from build123d import *

# Parameters (mm, degrees)
SKETCH1_R           = 2
SKETCH1_W           = 5
SKETCH1_H           = 5
BOSS_EXTRUDE7_DEPTH = 5
FILLET2_R           = 3


with BuildPart() as part:
    # Sketch1 → Boss-Extrude7 (new body)
    with BuildSketch(Plane(origin=(0, 0, 0), x_dir=(1, 0, 0), z_dir=(0, 1, 0))):
        Polygon((-29.056186132, 30.501621615), (-21.556186132, 30.501621615), (-21.556186132, 35.501621615), (-16.556186132, 35.501621615), (-16.556186132, 30.501621615), (-13.556186132, 30.501621615), (-13.556186132, 27.501621615), (-15.056186132, 27.501621615), (-15.056186132, 25.001621615), (-13.556186132, 25.001621615), (-13.556186132, 20.501621615), (-9.556186132, 20.501621615), (-9.556186132, 25.001621615), (-8.056186132, 25.001621615), (-8.056186132, 27.501621615), (-9.556186132, 27.501621615), (-9.556186132, 30.501621615), (-6.556186132, 30.501621615), (-6.556186132, 35.501621615), (-1.556186132, 35.501621615), (-1.556186132, 30.501621615), (5.943813868, 30.501621615), (5.943813868, -74.498378385), (-29.056186132, -74.498378385), align=None)
        with Locations(Location((0.443813868, 10.501621615, 0), (0, 0, 270))):
            Circle(SKETCH1_R, mode=Mode.SUBTRACT)
        with Locations(Location((-23.556186132, 10.501621615, 0), (0, 0, 90))):
            Circle(SKETCH1_R, mode=Mode.SUBTRACT)
        with Locations(Location((0.443813868, -46.498378385, 0), (0, 0, 90))):
            Circle(SKETCH1_R, mode=Mode.SUBTRACT)
        with Locations(Location((-23.556186132, -46.498378385, 0), (0, 0, 270))):
            Circle(SKETCH1_R, mode=Mode.SUBTRACT)
        with Locations(Location((-11.556186132, -68.998378385, 0), (0, 0, 270))):
            Circle(SKETCH1_R, mode=Mode.SUBTRACT)
        with Locations((-23.556186132, 3.001621615)):
            Rectangle(SKETCH1_W, SKETCH1_H, mode=Mode.SUBTRACT)
        with Locations((-23.556186132, 18.001621615)):
            Rectangle(SKETCH1_W, SKETCH1_H, mode=Mode.SUBTRACT)
        with Locations((0.443813868, 3.001621615)):
            Rectangle(SKETCH1_W, SKETCH1_H, mode=Mode.SUBTRACT)
        with Locations((0.443813868, 18.001621615)):
            Rectangle(SKETCH1_W, SKETCH1_H, mode=Mode.SUBTRACT)
        with Locations((0.443813868, -38.998378385)):
            Rectangle(SKETCH1_W, SKETCH1_H, mode=Mode.SUBTRACT)
        with Locations((0.443813868, -53.998378385)):
            Rectangle(SKETCH1_W, SKETCH1_H, mode=Mode.SUBTRACT)
        with Locations((-23.556186132, -53.998378385)):
            Rectangle(SKETCH1_W, SKETCH1_H, mode=Mode.SUBTRACT)
        with Locations((-23.556186132, -38.998378385)):
            Rectangle(SKETCH1_W, SKETCH1_H, mode=Mode.SUBTRACT)
        with Locations((-19.056186132, -68.998378385)):
            Rectangle(SKETCH1_W, SKETCH1_H, mode=Mode.SUBTRACT)
        with Locations((-4.056186132, -68.998378385)):
            Rectangle(SKETCH1_W, SKETCH1_H, mode=Mode.SUBTRACT)
    extrude(amount=BOSS_EXTRUDE7_DEPTH)

    # Fillet2
    fillet2_edges = [part.edges().sort_by_distance(p)[0] for p in [
        (5.943813868, 2.5, 74.498378385),
        (-29.056186132, 2.5, 74.498378385),
    ]]
    fillet(fillet2_edges, radius=FILLET2_R)


solid = part.part
Verification items for the finished model (mm, model axes). A direction names the side the tool comes from. Give positions to 0.01 mm unless a question says otherwise; leave off trailing zeros. Write each loop counter-clockwise with the first axis right and the second up, starting at its lowest first coordinate (ties: lowest second). Pieces come first, ordered by that corner, then holes. Notation, with made-up numbers: M 37,-19 L 61,-19 A22 ccw 61,20 Z; hole C -22.5,72.5 d2. An arc over 180 degrees is marked long. Put each result on its own line as item: value. Start each with the question number.
1. Scan lines: line 1 along Z through (x, y) = (-26, 1.7); line 2 along X through (y, z) = (1.85, -5); line 3 along Z through (x, y) = (-6.5, 0.75). Record each from-to range of solid material in increasing order. Write a range as [from, to].
2. Draft check along X on faces 4 (the face through (-25, 2, -30.502)), 5 (the face through (-21.556, 2, -33)), 6 (the face through (-26.056, 2, -3)). Enter one of: +X half, -X half, draft (parallel to the pull), parting line (faces both ways), or undercut.
3. Set-up check for faces 1 (the face through (-4, 2, -35.502)), 2 (the face through (-12, 2, -20.502)), 3 (the face through (-24, 2, -20.502)): record each of +Z, -Z, +X, -X, +Y, -Y from which the full face is reachable in a straight line by a thin tool's end or side.
4. Go/stop test with flat-tipped pins: pin 1 Ø2.5 at (x, y) = (-8.5, 2.5) entering from -Z; pin 2 Ø1.2 at (x, y) = (-11, 3.5) entering from -Z. Record where each tip stops, or that it passes through.
5. Section check A-A (z = 38.5). Record the cut outline in (x, y).
6. Section check B-B (y = 3.95). Give the number of separate pieces and of enclosed holes in the cut face, and give its area (3 significant figures).
Answer list:
1. line 1: [-30.5, -20.5], [-15.5, -5.5], [-0.5, 36.5], [41.5, 51.5], [56.5, 74.5]
1. line 2: [-29.06, -26.06], [-21.06, -2.06], [2.94, 5.94]
1. line 3: [-35.5, 66.5], [71.5, 74.5]
2. face 4: draft
2. face 5: -X half
2. face 6: undercut
3. face 1: -Z, +X, -X, +Y, -Y
3. face 2: -Z, +Y, -Y
3. face 3: +Y, -Y
4. pin 1: z = -30.5
4. pin 2: z = -20.5
5. outline: M -29.06,0 L -26.06,0 L -26.06,5 L -29.06,5 Z; M -21.06,0 L -2.06,0 L -2.06,5 L -21.06,5 Z; M 2.94,0 L 5.94,0 L 5.94,5 L 2.94,5 Z
6. separate pieces: 1
6. enclosed holes: 15
6. area: 3,360 mm2
